Part model, mm, in its own coordinate system. A direction names the side the tool comes from. Give positions to 0.01 mm unless a question says otherwise; leave off trailing zeros. Order: outer loops, then holes, each group sorted by start corner. A loop starts at its lowest first (then second) coordinate and runs counter-clockwise, first axis right, second up. Notation, with made-up numbers: M 63,47.25 L 87,47.25 A18 cw 87,77.25 Z; hole C 76,86.5 d5. An arc over 180 degrees is marked long. Return JSON: item names as keys, results as strings.
from build123d import *

# Parameters (mm, degrees)
SKETCH_1_W         = 54
SKETCH_1_H         = 29
EXTRUDE_1_DEPTH    = 1
EXTRUDE_2_DEPTH    = 1
EXTRUDE_3_DEPTH    = 1
SKETCH_4_W         = 1
SKETCH_4_H         = 20
EXTRUDE_4_DEPTH    = 8
SKETCH_5_W         = 1
SKETCH_5_H         = 20
EXTRUDE_5_DEPTH    = 8
SKETCH_6_W         = 21
SKETCH_6_H         = 1
EXTRUDE_6_DEPTH    = 20
HOLE_WIZARD_M3_1_D = 2.5
CHAMFER_1_SIZE     = 5
FILLET_1_R         = 0.5
FILLET_2_R         = 5
HOLE_WIZARD_M3_2_D = 2.5


with BuildPart() as part:
    # 草图1 → 凸台-拉伸1 (new body)
    with BuildSketch(Plane(origin=(0, 0, 0), x_dir=(1, 0, 0), z_dir=(0, 1, 0))):
        with Locations((-27, 14.5)):
            Rectangle(SKETCH_1_W, SKETCH_1_H)
    extrude(amount=EXTRUDE_1_DEPTH)

    # 草图2 → 凸台-拉伸2 (add)
    with BuildSketch(Plane.ZY.offset(54)):
        Polygon((-29, 0), (0, 0), (0, -20), align=None)
    extrude(amount=-EXTRUDE_2_DEPTH)

    # 草图3 → 凸台-拉伸3 (add)
    with BuildSketch(Plane(origin=(0, 0, 0), x_dir=(0, 0, -1), z_dir=(1, 0, 0))):
        Polygon((0, 0), (0, -20), (29, 0), align=None)
    extrude(amount=-EXTRUDE_3_DEPTH)

    # 草图4 → 凸台-拉伸4 (add)
    with BuildSketch(Plane.ZY.offset(1)):
        with Locations((-0.5, -10)):
            Rectangle(SKETCH_4_W, SKETCH_4_H)
    extrude(amount=EXTRUDE_4_DEPTH)

    # 草图5 → 凸台-拉伸5 (add)
    with BuildSketch(Plane(origin=(-53, 0, 0), x_dir=(0, 0, -1), z_dir=(1, 0, 0))):
        with Locations((0.5, -10)):
            Rectangle(SKETCH_5_W, SKETCH_5_H)
    extrude(amount=EXTRUDE_5_DEPTH)

    # 草图6 → 凸台-拉伸6 (add)
    with BuildSketch(Plane.XZ):
        with Locations((-18.5, -28.5)):
            Rectangle(SKETCH_6_W, SKETCH_6_H)
    extrude(amount=EXTRUDE_6_DEPTH)

    # M3 螺纹孔1 (through all)
    with Locations(Plane(origin=(0, 0, -29), x_dir=(-1, 0, 0), z_dir=(0, 0, -1))):
        with Locations((18, -10)):
            Hole(HOLE_WIZARD_M3_1_D / 2)

    # 倒角1
    chamfer_1_edges = [part.edges().sort_by_distance(p)[0] for p in [
        (-8, -20, -28.5),
        (-29, -20, -28.5),
    ]]
    chamfer(chamfer_1_edges, length=CHAMFER_1_SIZE)

    # 圆角1
    fillet_1_edges = [part.edges().sort_by_distance(p)[0] for p in [
        (-54, 1, -14.5),
        (0, 1, -14.5),
        (-27, 1, -29),
        (0, -9.5, 0),
        (-54, -9.5, 0),
    ]]
    fillet(fillet_1_edges, radius=FILLET_1_R)

    # 圆角2
    fillet_2_edges = [part.edges().sort_by_distance(p)[0] for p in [
        (-9, -20, -0.5),
        (-45, -20, -0.5),
    ]]
    fillet(fillet_2_edges, radius=FILLET_2_R)

    # M3 螺纹孔2 (through all)
    with Locations(Plane(origin=(0, 1, 0), x_dir=(1, 0, 0), z_dir=(0, 1, 0))):
        with Locations((-51, 22), (-51, 7), (-3.5, 7), (-3.5, 22)):
            Hole(HOLE_WIZARD_M3_2_D / 2)


solid = part.part
Q1. Band-saw the part on B-B (y = -10). Give the cut face in (x, z), then the cut area to 3 significant figures.
Established:
{"outline": "M -54,-14.5 L -53,-14.5 L -53,-1 L -45,-1 L -45,0 L -53.5,0 A0.5 ccw -54,-0.5 Z; M -29,-29 L -19.25,-29 L -19.25,-28 L -29,-28 Z; M -16.75,-29 L -8,-29 L -8,-28 L -16.75,-28 Z; M -9,-1 L -1,-1 L -1,-14.5 L 0,-14.5 L 0,-0.5 A0.5 ccw -0.5,0 L -9,0 Z", "area": "63.4 mm²"}
Q2. Band-saw the part on A-A (x = -51). Give the cut face in (y, z), then the cut area to 3 significant figures.
Established:
{"outline": "M -20,-1 L 0,-1 L 0,-5.75 L 1,-5.75 L 1,0 L -20,0 Z; M 0,-29 L 0.5,-29 A0.5 ccw 1,-28.5 L 1,-23.25 L 0,-23.25 Z; M 0,-20.75 L 1,-20.75 L 1,-8.25 L 0,-8.25 Z", "area": "43.9 mm²"}
Q3. Probe line 1 along Z through (x, y) = (-51, 0.25); line 2 along X through (y, z) = (-0.75, -23); line 3 along Z through (x, y) = (-22, -18). List the from-to ranges inside material, lowest first.
Established:
{"line 1": "z = -29 to -23.25, -20.75 to -8.25, -5.75 to 0", "line 2": "x = -54 to -53, -1 to 0", "line 3": "z = -29 to -28"}
Q4. Band-saw the part on D-D (y = -16.25). Give the cut face in (x, z), then the cut area to 3 significant figures.
Established:
{"outline": "M -54,-5.44 L -53,-5.44 L -53,-1 L -45.16,-1 L -45.16,0 L -53.5,0 A0.5 ccw -54,-0.5 Z; M -27.75,-29 L -9.25,-29 L -9.25,-28 L -27.75,-28 Z; M -8.84,-1 L -1,-1 L -1,-5.44 L 0,-5.44 L 0,-0.5 A0.5 ccw -0.5,0 L -8.84,0 Z", "area": "45.0 mm²"}
Q5. Band-saw the part on C-C (z = -7). Give the cut face in (x, y), then the cut area to 3 significant figures.
Established:
{"outline": "M -54,-15.17 L -53,-15.17 L -53,0 L -52.25,0 L -52.25,1 L -53.5,1 A0.5 ccw -54,0.5 Z; M -49.75,0 L -4.75,0 L -4.75,1 L -49.75,1 Z; M -2.25,0 L -1,0 L -1,-15.17 L 0,-15.17 L 0,0.5 A0.5 ccw -0.5,1 L -2.25,1 Z", "area": "79.2 mm²"}
Q6. 3-axis set-ups, long thin cutter, end or side, ignore diameter. For faces 1 (the flat face through (-51.5, -20, -0.5)), 2 (the cylindrical face through (-46.43, -18.5, -0.51)), 3 (the flat face through (-1, -7, -12)): which of +Z, -Z, +X, -X, +Y, -Y reach the whole face in a straight line?
Established:
{"face 1": "+Z, -Z, +X, -X, -Y", "face 2": "+Z, -Z, -Y", "face 3": "-Z, -Y"}
Q7. Pin check, flat tips, straight feed: pin 1 (6 mm diameter, centred on x = -16.5, y = -7, fed in from +Z); pin 2 (6 mm diameter, centred on x = -42.5, z = -12, fed in from -Y); pin 3 (0.8 mm diameter, centred on y = -5.5, z = -28.5, fed in from +X). Stop position of each tip, or through.
Established:
{"pin 1": "stops at z = -28", "pin 2": "stops at y = 0", "pin 3": "stops at x = -8"}
Q8. Two-plate mould, pull along Z, no slides. Class faces 4 (the flat face through (-27.1, 0.6, 0)), 5 (the flat face through (0, -7, -11)), 6 (the cylindrical face through (-51.577, 0.493, -5.891)), 7 (the flat face through (-53.51, -10.14, -14.3)): +Z half, -Z half, draft (parallel to the pull), parting line (faces both ways), or undercut.
Established:
{"face 4": "+Z half", "face 5": "draft", "face 6": "undercut", "face 7": "-Z half"}
